Answer from the drawing. Dimensions are ordinates in mm from the lowest x, y and z of the part. Round coordinates to 2 decimals unless told otherwise and drop trailing zeros. Write each loop counter-clockwise with the first axis right and the second up, starting at its lowest first coordinate (ties: lowest second). Pieces come first, ordered by that corner, then holes.
1. Find section B-B (y = 76.2). Count the separate pieces of the cut face and the enclosed holes in it, and give its area (3 significant figures).
2. Find section A-A (x = 292). Write down the section's boundary in (y, z), and give its area (3 significant figures).
3. Straight lines are drawn through the part: probe 1 along X at (y, z) = (78, 8) (1 decimal); probe 2 along X at (y, z) = (73, 12.75) (1 decimal); probe 3 along Y at (x, z) = (274, 11.5). For each, find the intervals that lie inside material, in ascending order.
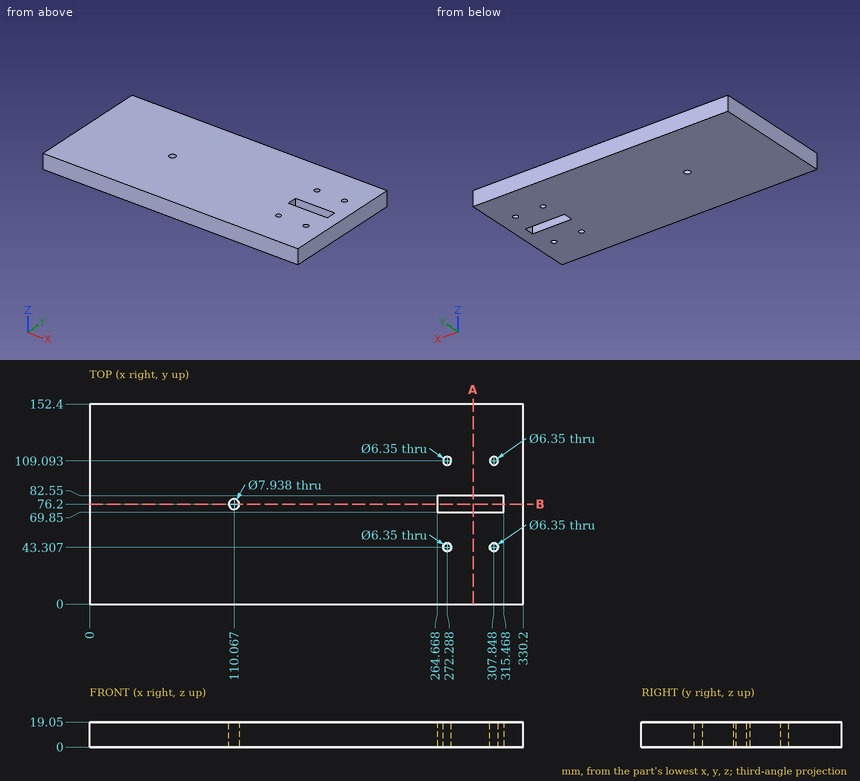
Worked answers:
1. separate pieces: 3
1. enclosed holes: 0
1. area: 5,170 mm2
2. outline: (0, 0) - (69.85, 0) - (69.85, 19.05) - (0, 19.05) - close; (82.55, 0) - (152.4, 0) - (152.4, 19.05) - (82.55, 19.05) - close
2. area: 2,660 mm2
3. probe 1: x = 0 to 106.5, 113.6 to 264.7, 315.5 to 330.2
3. probe 2: x = 0 to 107.7, 112.4 to 264.7, 315.5 to 330.2
3. probe 3: y = 0 to 40.63, 45.98 to 69.85, 82.55 to 106.42, 111.77 to 152.4
